```python
from build123d import *

# Parameters (mm, degrees)
F0_R        = 11.15
F0_R_2      = 11.35
F1_DEPTH    = 7
F2_C1_SIZE  = 1
F2_C2_SIZE  = 1
F2_C3_SIZE  = 1
F2_C4_SIZE  = 1
F2_C5_SIZE  = 1
F2_C6_SIZE  = 1
F2_C7_SIZE  = 0.9999
F2_C8_SIZE  = 0.9999
F2_C9_SIZE  = 0.9999
F2_C10_SIZE = 0.9999
F2_C11_SIZE = 0.9999
F2_C12_SIZE = 0.9999


# Not quite as in the source:
# - a fillet or chamfer is up to 0.001 mm smaller than in the source, because OpenCascade refuses the exact size


with BuildPart() as f1:
    # F0 (on Top) → F1 (new body)
    with BuildSketch(Plane.XY):
        with BuildLine():
            ThreePointArc((21.4042818528, 0), (11.7146810466, 7.3545646083), (11.3361036393, 19.5132924821))
            ThreePointArc((11.3361036393, 19.5132924821), (-0.5821803149, 39.3148759845), (-10.7021409264, 18.5366518343))
            ThreePointArc((-10.7021409264, 18.5366518343), (-12.2265803079, 6.4679290794), (-22.5670588206, 0.0607074905))
            ThreePointArc((-22.5670588206, 0.0607074905), (-33.7565911918, -20.1616209346), (-10.7021409264, -18.5366518343))
            ThreePointArc((-10.7021409264, -18.5366518343), (0.5118992613, -13.8224936877), (11.2309551813, -19.5739999726))
            ThreePointArc((11.2309551813, -19.5739999726), (34.3387715067, -19.15325505), (21.4042818528, 0))
        make_face()
        with Locations((-22.6706134247, -13.0888847634)):
            Circle(F0_R, mode=Mode.SUBTRACT)
        with BuildLine():
            ThreePointArc((-11.9684724983, -5.4477670709), (-11.2823793649, -6.5138847634), (-10.7021409264, -7.6411176926))
            ThreePointArc((-10.7021409264, -7.6411176926), (-11.3882340598, -6.575), (-11.9684724983, -5.4477670709))
        make_face(mode=Mode.SUBTRACT)
        with Locations((22.6706134247, -13.0888847634)):
            Circle(F0_R, mode=Mode.SUBTRACT)
        with BuildLine():
            ThreePointArc((11.9684724983, -5.4477670709), (11.3882340598, -6.575), (10.7021409264, -7.6411176926))
            ThreePointArc((10.7021409264, -7.6411176926), (11.2823793649, -6.5138847634), (11.9684724983, -5.4477670709))
        make_face(mode=Mode.SUBTRACT)
        Circle(F0_R_2, mode=Mode.SUBTRACT)
        with BuildLine():
            ThreePointArc((-1.2663315719, 13.0888847634), (0, 13.15), (1.2663315719, 13.0888847634))
            ThreePointArc((1.2663315719, 13.0888847634), (0, 13.0277695268), (-1.2663315719, 13.0888847634))
        make_face(mode=Mode.SUBTRACT)
        with Locations((0, 26.1777695268)):
            Circle(F0_R, mode=Mode.SUBTRACT)
    extrude(amount=F1_DEPTH)

    # F2: chamfer of 1 on 12 edges, made by hand

    # F2_c1
    f2_c1_edges = [f1.edges().sort_by_distance(p)[0] for p in [
        (0.5118992613, -13.8224936877, 0),
    ]]
    chamfer(f2_c1_edges, length=F2_C1_SIZE)

    # F2_c2
    f2_c2_edges = [f1.edges().sort_by_distance(p)[0] for p in [
        (0.5118992613, -13.8224936877, 7),
    ]]
    chamfer(f2_c2_edges, length=F2_C2_SIZE)

    # F2_c3
    f2_c3_edges = [f1.edges().sort_by_distance(p)[0] for p in [
        (11.7146810466, 7.3545646083, 0),
    ]]
    chamfer(f2_c3_edges, length=F2_C3_SIZE)

    # F2_c4
    f2_c4_edges = [f1.edges().sort_by_distance(p)[0] for p in [
        (11.7146810466, 7.3545646083, 7),
    ]]
    chamfer(f2_c4_edges, length=F2_C4_SIZE)

    # F2_c5
    f2_c5_edges = [f1.edges().sort_by_distance(p)[0] for p in [
        (-12.2265803079, 6.4679290794, 0),
    ]]
    chamfer(f2_c5_edges, length=F2_C5_SIZE)

    # F2_c6
    f2_c6_edges = [f1.edges().sort_by_distance(p)[0] for p in [
        (-12.2265803079, 6.4679290794, 7),
    ]]
    chamfer(f2_c6_edges, length=F2_C6_SIZE)

    # F2_c7 (size 1 in the source; OpenCascade refuses exactly that, so slightly less here)
    f2_c7_edges = [f1.edges().sort_by_distance(p)[0] for p in [
        (-33.7565911918, -20.1616209346, 0),
    ]]
    chamfer(f2_c7_edges, length=F2_C7_SIZE)

    # F2_c8 (size 1 in the source; OpenCascade refuses exactly that, so slightly less here)
    f2_c8_edges = [f1.edges().sort_by_distance(p)[0] for p in [
        (-33.7565911918, -20.1616209346, 7),
    ]]
    chamfer(f2_c8_edges, length=F2_C8_SIZE)

    # F2_c9 (size 1 in the source; OpenCascade refuses exactly that, so slightly less here)
    f2_c9_edges = [f1.edges().sort_by_distance(p)[0] for p in [
        (34.3387715067, -19.15325505, 0),
    ]]
    chamfer(f2_c9_edges, length=F2_C9_SIZE)

    # F2_c10 (size 1 in the source; OpenCascade refuses exactly that, so slightly less here)
    f2_c10_edges = [f1.edges().sort_by_distance(p)[0] for p in [
        (34.3387715067, -19.15325505, 7),
    ]]
    chamfer(f2_c10_edges, length=F2_C10_SIZE)

    # F2_c11 (size 1 in the source; OpenCascade refuses exactly that, so slightly less here)
    f2_c11_edges = [f1.edges().sort_by_distance(p)[0] for p in [
        (-0.5821803149, 39.3148759845, 0),
    ]]
    chamfer(f2_c11_edges, length=F2_C11_SIZE)

    # F2_c12 (size 1 in the source; OpenCascade refuses exactly that, so slightly less here)
    f2_c12_edges = [f1.edges().sort_by_distance(p)[0] for p in [
        (-0.5821803149, 39.3148759845, 7),
    ]]
    chamfer(f2_c12_edges, length=F2_C12_SIZE)


solid = f1.part
```
Can you work these out from the model? Positions are in its coordinate system, mm. Give positions to 0.01 mm unless a question says otherwise; leave off trailing zeros. Loops run counter-clockwise (first coordinate to the right, second up) from the corner with the lowest first, then second, coordinate; pieces in that order, holes last. Notation, with made-up numbers: M 35.5,-14 L 78.5,-14 A22 cw 78.5,21 Z; hole C -38.5,38 d10. An arc over 180 degrees is marked long. One line per question, with ' | ' between items. Start each with the question number.
Q1. For pin 1 Ø2 at (y, z) = (31, 1) entering from -X; pin 2 Ø1.5 at (x, z) = (17, 2) entering from +Y; pin 3 Ø2 at (x, z) = (4, 4) entering from -Y, each with a flat end and sliding along its axis, tell me the tip position at first contact or that it passes through.
Q2. If we mould it in two halves opening along X, with no side actions, what happens to faces 1 (the flat face through (0, -12, 7)), 2 (the cylindrical face through (-0.187, 39.326, 3.465)), 3 (the cylindrical face through (10.485, -4.347, 3.451))? For each: +X half, -X half, draft (parallel to the pull), parting line (faces both ways), or undercut.
Q3. If we section it at B-B (y = -15): State how many separate pieces and enclosed holes the cut face has, plus the area to 3 significant figures.
Q4. If we section it at A-A (z = 4.5): Please give me the cut outline in (x, y), plus the area to 3 significant figures.
Q5. If I drill on line 1 (X direction, y = -4, z = 3); line 2 (Y direction, x = -4.5, z = 6.25); line 3 (Y direction, x = -31.5, z = 3.75), over which ranges is the centre line in solid material (lowest first)? Write a range as from..to.
Computed:
1) pin 1: stops at x = -12.58 | pin 2: stops at y = 2.2 | pin 3: stops at y = -14.78
2) face 1: draft | face 2: parting line | face 3: undercut
3) separate pieces: 4 | enclosed holes: 0 | area: 106 mm²
4) outline: M -22.57,0.06 A13.15 ccw long -10.7,-18.54 A14.12 cw 11.23,-19.57 A13.15 ccw long 21.4,0 A14.12 cw 11.34,19.51 A13.15 ccw long -10.7,18.54 A14.12 cw Z; hole C -22.67,-13.09 d22.3; hole M -11.97,-5.45 A13.15 ccw -10.7,-7.64 A13.15 ccw Z; hole C 0,0 d22.7; hole C 0,26.18 d22.3; hole M -1.27,13.09 A13.15 ccw 1.27,13.09 A13.15 ccw Z; hole M 10.7,-7.64 A13.15 ccw 11.97,-5.45 A13.15 ccw Z; hole C 22.67,-13.09 d22.3 | area: 788 mm²
5) line 1: x = -32.17..-29.13, -16.21..-10.62, 10.62..16.21, 29.13..32.17 | line 2: y = -14.23..-10.42, 10.42..15.98, 36.38..38.27 | line 3: y = -22.83..-19.9, -6.28..-3.34
